Print and shaded views of the part. All mm, measured from the part's lowest x, y and z. A direction names the side the tool comes from. Give positions to 0.01 mm unless a question says otherwise; leave off trailing zeros. Loops run counter-clockwise (first coordinate to the right, second up) from the corner with the lowest first, then second, coordinate; pieces in that order, holes last. Notation, with made-up numbers: M 65,-16 L 104,-16 A21 ccw 104,7 Z; hole C 3.5,-8.75 d4. An arc over 180 degrees is marked long. Answer in a Markdown table with one row per item.
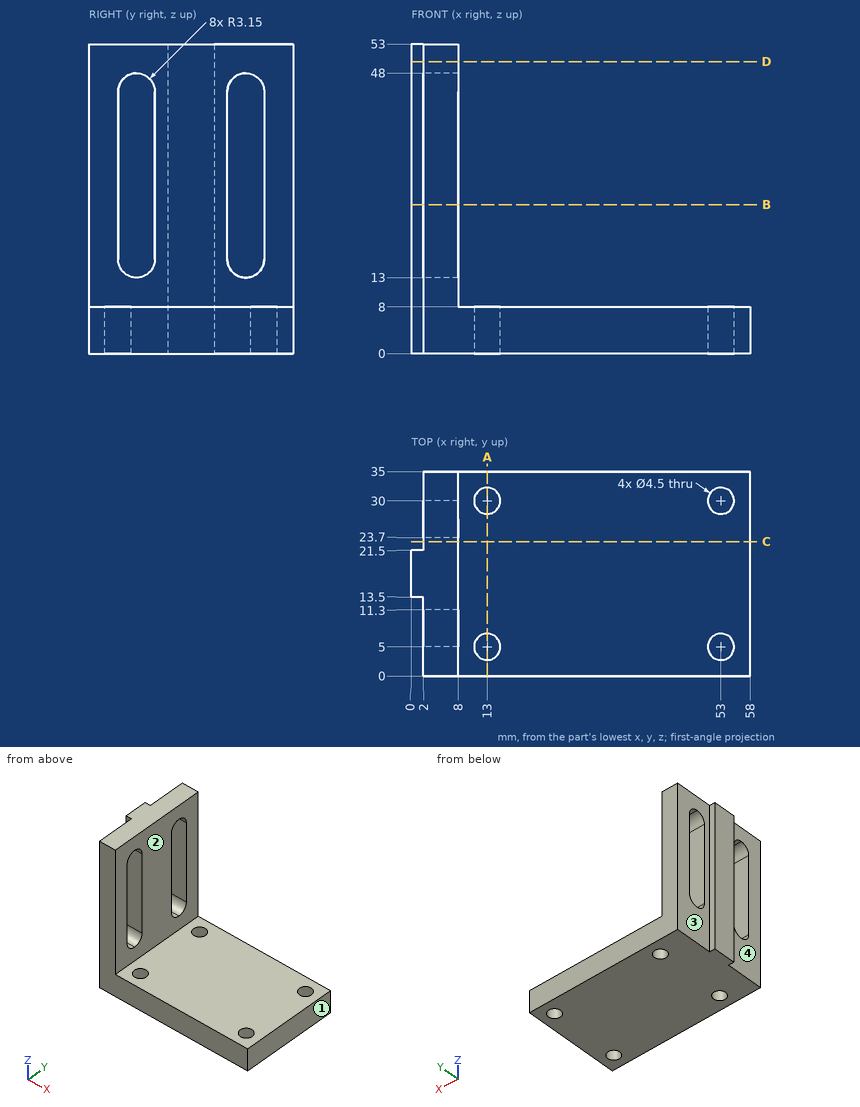
(1) Which spindle directions (+Z, -Z, +X, -X, +Y, -Y) get a long thin tool onto all of the face, cutting with end or side? Do the marked faces 1, 2, 3 and 4. Say none if no direction does.
Established:
| item | result |
|---|---|
| face 1 | +Z, -Z, +X, +Y, -Y |
| face 2 | +Z, +X, +Y, -Y |
| face 3 | +Z, -Z, -X, +Y |
| face 4 | +Z, -Z, -X, -Y |
(2) Saw through at C-C, the plane y = 23. Give the cut face in (x, z), and give its area (3 significant figures).
Established:
| item | result |
|---|---|
| outline | M 2,0 L 58,0 L 58,8 L 8,8 L 8,53 L 2,53 Z |
| area | 718 mm2 |
(3) Saw through at A-A, the plane x = 13. Give the cut face in (y, z), and give its area (3 significant figures).
Established:
| item | result |
|---|---|
| outline | M 0,0 L 2.75,0 L 2.75,8 L 0,8 Z; M 7.25,0 L 27.75,0 L 27.75,8 L 7.25,8 Z; M 32.25,0 L 35,0 L 35,8 L 32.25,8 Z |
| area | 208 mm2 |
(4) Saw through at B-B, the plane z = 25.5. Give the cut face in (x, y), and give its area (3 significant figures).
Established:
| item | result |
|---|---|
| outline | M 0,13.5 L 2,13.5 L 2,11.3 L 8,11.3 L 8,23.7 L 2,23.7 L 2,21.5 L 0,21.5 Z; M 2,0 L 8,0 L 8,5 L 2,5 Z; M 2,30 L 8,30 L 8,35 L 2,35 Z |
| area | 150 mm2 |
(5) Wall check: L1, parallel to X at y = 30, z = 5; L2, parallel to Y at x = 53, z = 6; L3, parallel to X at y = 32, z = 3.5. Give the ranges that are in metal, low to high.
Established:
| item | result |
|---|---|
| L1 | x = 2 to 10.75, 15.25 to 50.75, 55.25 to 58 |
| L2 | y = 0 to 2.75, 7.25 to 27.75, 32.25 to 35 |
| L3 | x = 2 to 11.97, 14.03 to 51.97, 54.03 to 58 |
(6) Saw through at D-D, the plane z = 50. Give the cut face in (x, y).
Established:
| item | result |
|---|---|
| outline | M 0,13.5 L 2,13.5 L 2,0 L 8,0 L 8,35 L 2,35 L 2,21.5 L 0,21.5 Z |
(7) Flat gauge pins, fed straight in: P1, Ø0.6, axis at x = 1, z = 22, coming from the +Y side; P2, Ø3, axis at y = 24, z = 34.5, coming from the +X side; P3, Ø1.5, axis at y = 29, z = 8.5, coming from the -X side. Where does each tip first touch, or does it go through?
Established:
| item | result |
|---|---|
| P1 | stops at y = 21.5 |
| P2 | stops at x = 8 |
| P3 | stops at x = 2 |
